from build123d import *

# Parameters (mm, degrees)
SKETCH_1_W          = 42
SKETCH_1_H          = 50
EXTRUDE_1_DEPTH     = 3
SKETCH_3_W          = 3
SKETCH_3_H          = 5
SKETCH_3_H_2        = 10
EXTRUDE_2_DEPTH     = 12
FILLET_1_R          = 5
FILLET_2_R          = 5
SKETCH_4_R          = 1
CUT_EXTRUDE_1_DEPTH = 27
SKETCH_5_R          = 2.5
EXTRUDE_3_DEPTH     = 3
SKETCH_6_W          = 9
SKETCH_6_H          = 12.266046359
CUT_EXTRUDE_2_DEPTH = 4
SKETCH_7_R          = 1.65
CUT_EXTRUDE_3_DEPTH = 16
FILLET_3_R          = 3


with BuildPart() as part:
    # 草图1 → 凸台-拉伸1 (new body)
    with BuildSketch(Plane.XY):
        Rectangle(SKETCH_1_W, SKETCH_1_H)
    extrude(amount=EXTRUDE_1_DEPTH)

    # 草图3 → 凸台-拉伸2 (add)
    with BuildSketch(Plane(origin=(0, 0, 0), x_dir=(-1, 0, 0), z_dir=(0, 0, -1))):
        with Locations((3.5, -22.5)):
            Rectangle(SKETCH_3_W, SKETCH_3_H)
        with Locations((3.5, 8)):
            Rectangle(SKETCH_3_W, SKETCH_3_H_2)
    extrude(amount=EXTRUDE_2_DEPTH)

    # 圆角1
    fillet_1_edges = [part.edges().sort_by_distance(p)[0] for p in [
        (-2, 8, 0),
    ]]
    fillet(fillet_1_edges, radius=FILLET_1_R)

    # 圆角2
    fillet_2_edges = [part.edges().sort_by_distance(p)[0] for p in [
        (-2, -22.5, 0),
    ]]
    fillet(fillet_2_edges, radius=FILLET_2_R)

    # 草图4 → 切除-拉伸1 (cut, through all)
    with BuildSketch(Plane.ZY.offset(5)):
        with Locations((-5.946968178, -22)):
            Circle(SKETCH_4_R)
        with Locations((-5.946968178, 5)):
            Circle(SKETCH_4_R)
    extrude(amount=-CUT_EXTRUDE_1_DEPTH, mode=Mode.SUBTRACT)

    # 草图5 → 凸台-拉伸3 (add)
    with BuildSketch(Plane(origin=(21, 0, 0), x_dir=(0, 0, -1), z_dir=(1, 0, 0))):
        with BuildLine():
            Line((0, -4.733953641), (0, -12.733953641))
            Line((0, -12.733953641), (3.333333333, -15.715377611))
            ThreePointArc((3.333333333, -15.715377611), (9.249103106, -15.067047939), (7.972848445, -9.254317307))
            Line((7.972848445, -9.254317307), (0, -4.733953641))
        make_face()
        with Locations((6, -12.733953641)):
            Circle(SKETCH_5_R, mode=Mode.SUBTRACT)
    extrude(amount=-EXTRUDE_3_DEPTH)

    # 草图6 → 切除-拉伸2 (cut, through all)
    with BuildSketch(Plane(origin=(0, 0, 0), x_dir=(-1, 0, 0), z_dir=(0, 0, -1))):
        with Locations((-16.5, -18.86697682)):
            Rectangle(SKETCH_6_W, SKETCH_6_H)
        with Locations((16.5, -18.86697682)):
            Rectangle(SKETCH_6_W, SKETCH_6_H)
    extrude(amount=-CUT_EXTRUDE_2_DEPTH, mode=Mode.SUBTRACT)

    # 草图7 → 切除-拉伸3 (cut, through all)
    with BuildSketch(Plane.XY.offset(3)):
        with Locations((9.975799492, 17.266046359)):
            Circle(SKETCH_7_R)
        with Locations((-10.024200508, 17.266046359)):
            Circle(SKETCH_7_R)
    extrude(amount=-CUT_EXTRUDE_3_DEPTH, mode=Mode.SUBTRACT)

    # 圆角3
    fillet_3_edges = [part.edges().sort_by_distance(p)[0] for p in [
        (-3.5, -25, -12),
    ]]
    fillet(fillet_3_edges, radius=FILLET_3_R)


solid = part.part
Could you check a few things on this model? Use its own coordinates, in mm. A direction names the side the tool comes from. Give positions to 0.01 mm unless a question says otherwise; leave off trailing zeros. Order: outer loops, then holes, each group sorted by start corner. A loop starts at its lowest first (then second) coordinate and runs counter-clockwise, first axis right, second up.
1. Suppose I cut it at B-B (z = -6). Write out the boundary of the cut face in (x, y), plus the area to 3 significant figures.
Answers below:
outline: (-5, -25) - (-2, -25) - (-2, -23) - (-5, -23) - close; (-5, -21) - (-2, -21) - (-2, -20) - (-5, -20) - close; (-5, 3) - (-2, 3) - (-2, 4) - (-5, 4) - close; (-5, 6) - (-2, 6) - (-2, 13) - (-5, 13) - close; (18, -16.73) - (21, -16.73) - (21, -15.23) - (18, -15.23) - close; (18, -10.23) - (21, -10.23) - (21, -8.14) - (18, -8.14) - close
area: 43.8 mm2
2. Which directions (+Z, -Z, +X, -X, +Y, -Y) give clear straight access to the entire face, cutting with the end or side of a thin tool? Please do faces 4 (the flat face through (-2, -23, -8)), 5 (the flat face through (-5, -24, -6)), 6 (the flat face through (-12, -19, 1)).
Answers below:
face 4: -Z, +X, +Y, -Y
face 5: -Z, -X, +Y, -Y
face 6: +Z, -Z, -X, -Y
3. I need wall thicknesses on L1, parallel to Z at x = -3, y = 5; L2, parallel to X at y = 16, z = 0.5; L3, parallel to Z at x = 11, y = 1.5. Which ranges of each line are inside material? Lowest first, please.
Answers below:
L1: z = -12 to -6.95, -4.95 to 3
L2: x = -21 to -11.08, -8.97 to 8.92, 11.03 to 21
L3: z = 0 to 3
4. Suppose I cut it at C-C (z = -2.5). Write out the boundary of the cut face in (x, y).
Answers below:
outline: (-5, -25) - (-1.33, -25) - (-1.33, -20) - (-5, -20) - close; (-5, 3) - (-1.33, 3) - (-1.33, 13) - (-5, 13) - close; (18, -14.97) - (21, -14.97) - (21, -6.15) - (18, -6.15) - close
5. Thinking about a two-plate mould opening in Y: for faces 1 (the cylindrical face through (19.521, -15.143, -9.193)), 2 (the cylindrical face through (-3.52, -22.89, -5.49)), 3 (the flat face through (-3, 8, -12)), which applies, +Y half, -Y half, draft (parallel to the pull), parting line (faces both ways), or undercut?
Answers below:
face 1: parting line
face 2: undercut
face 3: draft
6. Suppose I cut it at D-D (y = -18.5). Write out the boundary of the cut face in (x, z), plus the area to 3 significant figures.
Answers below:
outline: (-12, 0) - (12, 0) - (12, 3) - (-12, 3) - close
area: 72.0 mm2
7. For pin 1 (1.5 mm diameter, centred on y = -20.5, z = 1.5, fed in from +X); pin 2 (5.5 mm diameter, centred on y = 10, z = -7, fed in from +X); pin 3 (2.5 mm diameter, centred on y = -22, z = -5.95, fed in from -X), each with a flat end and sliding along its axis, tell me the tip position at first contact or that it passes through.
Answers below:
pin 1: stops at x = 12
pin 2: stops at x = -1.94
pin 3: stops at x = -5
8. Suppose I cut it at A-A (x = -4). Write out the boundary of the cut face in (y, z).
Answers below:
outline: (-25, -9) arc R3 ccw to (-22, -12) - (-20, -12) - (-20, 0) - (3, 0) - (3, -12) - (13, -12) - (13, 0) - (25, 0) - (25, 3) - (-25, 3) - close; hole circle Ø2 at (-22, -5.95); hole circle Ø2 at (5, -5.95)
